Geometry check sheet. Reference: the model listing, model coordinates, mm. Face numbers are marked on the shaded views. A direction names the side the tool comes from. Round coordinates to 2 decimals unless told otherwise and drop trailing zeros. Write each loop counter-clockwise with the first axis right and the second up, starting at its lowest first coordinate (ties: lowest second). Pieces come first, ordered by that corner, then holes. Notation, with made-up numbers: (-13, 3) -> (25, 3) arc R21 cw to (25, 10) -> close; hole circle Ø11 at (-36, -22.5). An arc over 180 degrees is marked (long way). Put each result on its own line as item: value. Start each with the question number.
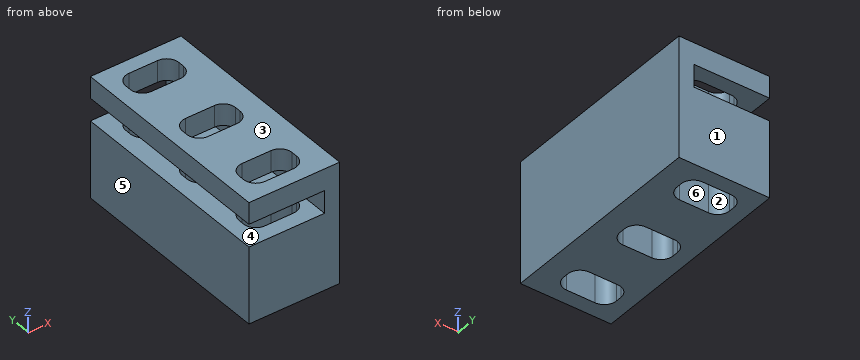
from build123d import *

# Parameters (mm, degrees)
F0_W     = 19.05
F0_H     = 44.45
F1_DEPTH = 25.4
F2_W     = 15.875
F2_H     = 4.7625
F2_W_2   = 9.525
F3_DEPTH = 45.974


with BuildPart() as f1:
    # F0 (on Top) → F1 (new body)
    with BuildSketch(Plane.XY):
        with Locations((0, -22.225)):
            Rectangle(F0_W, F0_H)
        with BuildLine():
            ThreePointArc((-6.35, -37.465), (-5.606051, -35.668949), (-3.81, -34.925))
            Line((-3.81, -34.925), (2.2225, -34.925))
            ThreePointArc((2.2225, -34.925), (4.018551, -35.668949), (4.7625, -37.465))
            Line((4.7625, -37.465), (4.7625, -38.735))
            ThreePointArc((4.7625, -38.735), (4.018551, -40.531051), (2.2225, -41.275))
            Line((2.2225, -41.275), (-3.81, -41.275))
            ThreePointArc((-3.81, -41.275), (-5.606051, -40.531051), (-6.35, -38.735))
            Line((-6.35, -38.735), (-6.35, -37.465))
        make_face(mode=Mode.SUBTRACT)
        with BuildLine():
            ThreePointArc((-6.35, -21.59), (-5.606051, -19.793949), (-3.81, -19.05))
            Line((-3.81, -19.05), (2.2225, -19.05))
            ThreePointArc((2.2225, -19.05), (4.018551, -19.793949), (4.7625, -21.59))
            Line((4.7625, -21.59), (4.7625, -22.86))
            ThreePointArc((4.7625, -22.86), (4.018551, -24.656051), (2.2225, -25.4))
            Line((2.2225, -25.4), (-3.81, -25.4))
            ThreePointArc((-3.81, -25.4), (-5.606051, -24.656051), (-6.35, -22.86))
            Line((-6.35, -22.86), (-6.35, -21.59))
        make_face(mode=Mode.SUBTRACT)
        with BuildLine():
            ThreePointArc((-6.35, -5.715), (-5.606051, -3.918949), (-3.81, -3.175))
            Line((-3.81, -3.175), (2.2225, -3.175))
            ThreePointArc((2.2225, -3.175), (4.018551, -3.918949), (4.7625, -5.715))
            Line((4.7625, -5.715), (4.7625, -6.985))
            ThreePointArc((4.7625, -6.985), (4.018551, -8.781051), (2.2225, -9.525))
            Line((2.2225, -9.525), (-3.81, -9.525))
            ThreePointArc((-3.81, -9.525), (-5.606051, -8.781051), (-6.35, -6.985))
            Line((-6.35, -6.985), (-6.35, -5.715))
        make_face(mode=Mode.SUBTRACT)
    extrude(amount=F1_DEPTH)

    # F2 (on face) → F3 (cut)
    with BuildSketch(Plane(origin=(0, 0, 0), x_dir=(-1, 0, 0), z_dir=(0, 1, 0))):
        with Locations((1.5875, 18.481419)):
            Rectangle(F2_W, F2_H)
        with Locations((14.2875, 18.481419)):
            Rectangle(F2_W_2, F2_H)
    extrude(amount=-F3_DEPTH, mode=Mode.SUBTRACT)


solid = f1.part
(1) Material ranges on L1, parallel to Y at x = 1, z = 24.25 (3 decimals); L2, parallel to Z at x = -2.5, y = -33; L3, parallel to Y at x = -5, z = 10.75, recorded low to high. Write a range as from..to.
(2) Sectioned sample at D-D (y = -11). Record the cut outline in (x, z) (3 decimals), and give its area (3 significant figures).
(3) Set-up check for the marked faces 4, 5 and 6: record each of +Z, -Z, +X, -X, +Y, -Y from which the full face is reachable in a straight line by a thin tool's end or side.
(4) Sectioned sample at B-B (z = 2.5). State how many separate pieces and enclosed holes the cut face has, and give its area (3 significant figures).
(5) Sectioned sample at A-A (x = 5.25). Record the cut outline in (y, z), and give its area (3 significant figures).
(6) Mould release check, pull along Y, two halves, no side actions. Record for the marked faces 1, 2 and 3: +Y half, -Y half, draft (parallel to the pull), parting line (faces both ways), or undercut.
Found:
1. L1: -44.45..-41.275, -34.925..-25.4, -19.05..-9.525, -3.175..0
1. L2: 0..16.1, 20.86..25.4
1. L3: -44.45..-40.98, -35.22..-25.1, -19.35..-9.23, -3.47..0
2. outline: (-9.525, 0) -> (9.525, 0) -> (9.525, 25.4) -> (-9.525, 25.4) -> (-9.525, 20.863) -> (6.35, 20.863) -> (6.35, 16.1) -> (-9.525, 16.1) -> close
2. area: 408 mm2
3. face 4: -X, +Y, -Y
3. face 5: +Z, -Z, -X, +Y, -Y
3. face 6: +Z, -Z
4. separate pieces: 1
4. enclosed holes: 3
4. area: 652 mm2
5. outline: (-44.45, 0) -> (0, 0) -> (0, 16.1) -> (-44.45, 16.1) -> close; (-44.45, 20.86) -> (0, 20.86) -> (0, 25.4) -> (-44.45, 25.4) -> close
5. area: 917 mm2
6. face 1: +Y half
6. face 2: undercut
6. face 3: draft
